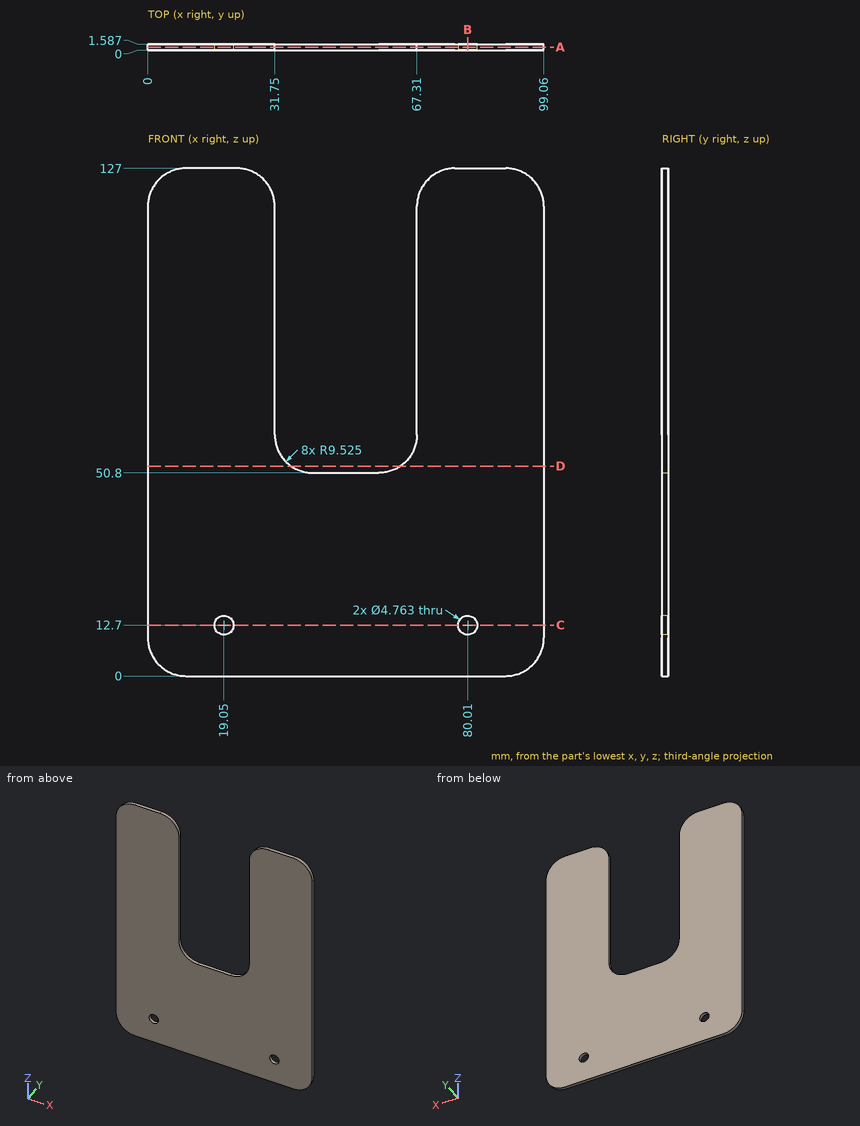
Here's the drawing with two shaded views (mm, measured from the low corner). I have some questions. Coordinates: 2 decimals unless noted, no trailing zeros. Order: outer loops, then holes, each group sorted by start corner. A loop starts at its lowest first (then second) coordinate and runs counter-clockwise, first axis right, second up.
Item 1: If we section it at D-D, the plane z = 52.5: List the corners of the cut face in (x, y) for me (1 decimal), then the cut area to 3 significant figures.
Response values:
outline: (0, 0) - (35.8, 0) - (35.8, 1.6) - (0, 1.6) - close; (63.2, 0) - (99.1, 0) - (99.1, 1.6) - (63.2, 1.6) - close
area: 114 mm2
Item 2: I need wall thicknesses on probe 1 along X at (y, z) = (0.6, 12.7); probe 2 along Z at (x, y) = (19.05, 1); probe 3 along X at (y, z) = (0.55, 75). Which ranges of each line are inside material? Lowest first, please.
Response values:
probe 1: x = 0 to 16.67, 21.43 to 77.63, 82.39 to 99.06
probe 2: z = 0 to 10.32, 15.08 to 127
probe 3: x = 0 to 31.75, 67.31 to 99.06
Item 3: If we section it at A-A, the plane y = 0.8: Give the number of separate pieces and of enclosed holes in the cut face, then the cut area to 3 significant figures.
Response values:
separate pieces: 1
enclosed holes: 2
area: 9,760 mm2
Item 4: If we section it at B-B, the plane x = 80.01: List the corners of the cut face in (y, z) for me.
Response values:
outline: (0, 0) - (1.59, 0) - (1.59, 10.32) - (0, 10.32) - close; (0, 15.08) - (1.59, 15.08) - (1.59, 127) - (0, 127) - close
Item 5: If we section it at C-C, the plane z = 12.7: List the corners of the cut face in (x, y) for me.
Response values:
outline: (0, 0) - (16.67, 0) - (16.67, 1.59) - (0, 1.59) - close; (21.43, 0) - (77.63, 0) - (77.63, 1.59) - (21.43, 1.59) - close; (82.39, 0) - (99.06, 0) - (99.06, 1.59) - (82.39, 1.59) - close
Item 6: I'm going to push a flat-ended pin straight in: pin 1 Ø2 at (x, z) = (86.5, 34.5) entering from -Y. Where does the tip first touch, or does it pass through?
Response values:
pin 1: stops at y = 0
